For this review, use the dimensioned drawing (mm, ordinates from the lowest corner) and the shaded views. Round coordinates to 2 decimals unless told otherwise and drop trailing zeros. Loops run counter-clockwise (first coordinate to the right, second up) from the corner with the lowest first, then second, coordinate; pieces in that order, holes last. Notation, with made-up numbers: (44, -36.75) - (98, -36.75) arc R15 cw to (98, -22.75) - close; hole circle Ø3 at (-35.5, -8.5). An arc over 180 degrees is marked (long way). Answer as CSV lines item,"result". Start each with the question number.
(1) Wall thickness on L1, parallel to X at y = 118, z = 0.85 (1 decimal); L2, parallel to Y at x = 216.5, z = 0.7; L3, parallel to X at y = 99.5, z = 1.75 (1 decimal): over which ranges is each line inside the solid? List them lowest first.
(2) For P1, Ø2, axis at x = 203.12, y = 82.55, coming from the +Z side; P2, Ø12, axis at x = 164, y = 77.5, coming from the -Z side, all flat-tipped, find the tip position at first contact; note any pin that passes through.
(3) Consider section B-B (y = 115.5). Give the boundary of the cut face in (x, z) (1 decimal).
(4) Consider section A-A (z = 2.1). Count the separate pieces of the cut face and the enclosed holes in it, and give its area (3 significant figures).
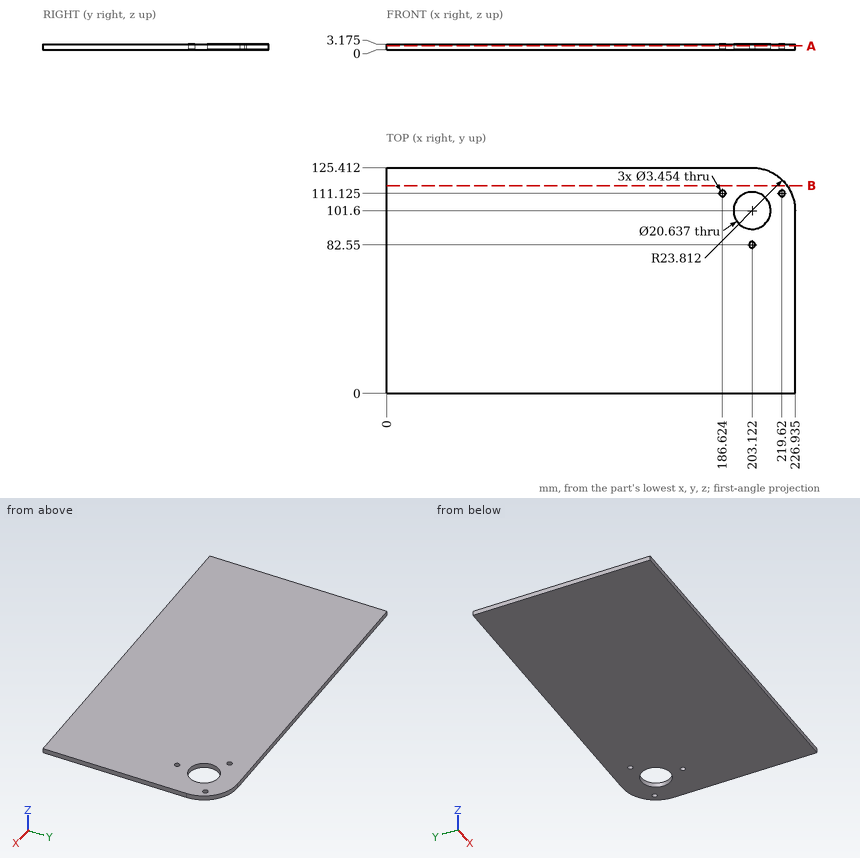
Determined:
1,L1,"x = 0 to 220.4"
1,L2,"y = 0 to 121.3"
1,L3,"x = 0 to 193, 213.2 to 226.9"
2,P1,"passes through"
2,P2,"stops at z = 0"
3,outline,"(0, 0) - (222.5, 0) - (222.5, 3.2) - (0, 3.2) - close"
4,separate pieces,"1"
4,enclosed holes,"4"
4,area,"28,000 mm^2"
